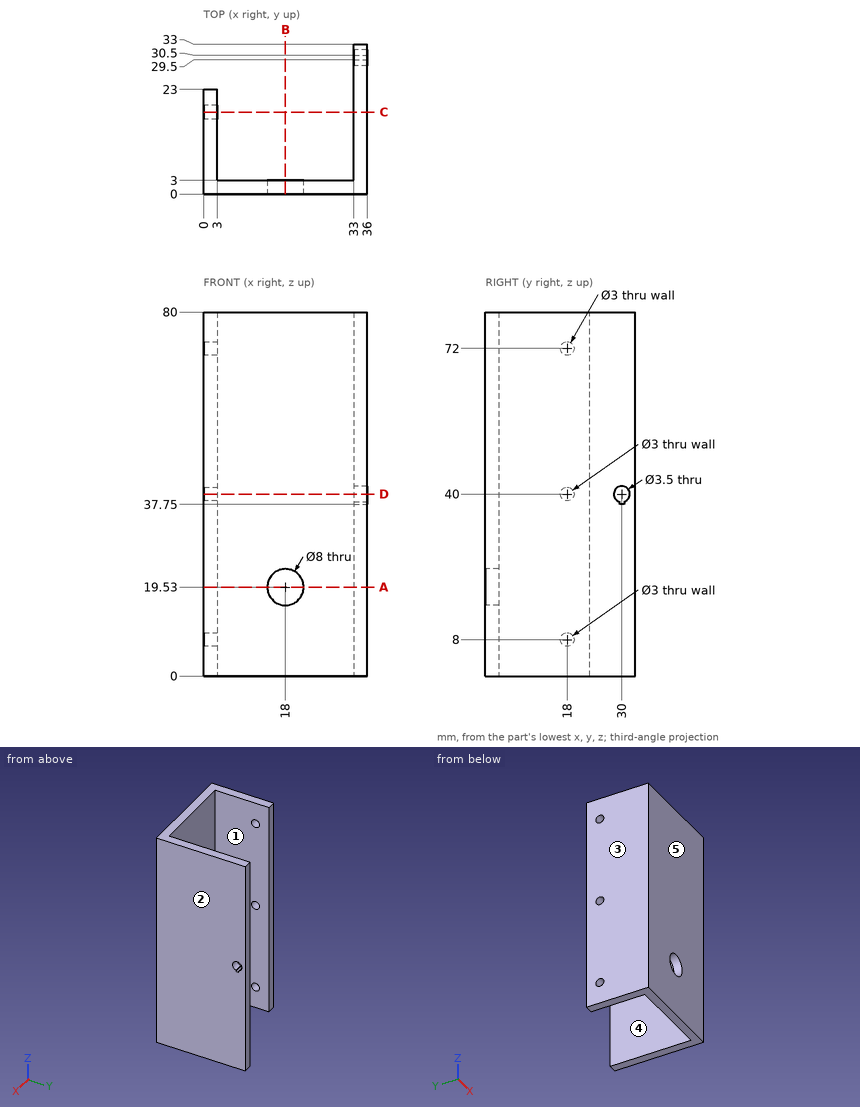
Source: three-view drawing plus pictorial views. Frame: mm from the lowest corner of the part. A direction names the side the tool comes from. Give positions to 0.01 mm unless a question says otherwise; leave off trailing zeros. Order: outer loops, then holes, each group sorted by start corner. A loop starts at its lowest first (then second) coordinate and runs counter-clockwise, first axis right, second up. Notation, with made-up numbers: (77.25, -28) - (106.25, -28) arc R18 ccw to (106.25, 5) - close; hole circle Ø3 at (-28.75, 0.5). An arc over 180 degrees is marked (long way). Put each result on its own line as item: value.
Item 1: Ray query, L1, parallel to X at y = 12, z = 74; L2, parallel to Y at x = 0.95, z = 40; L3, parallel to Z at x = 18, y = 2. Return the intervals inside material, ascending. Write a range as from..to.
Found:
L1: x = 0..3, 33..36
L2: y = 0..16.5, 19.5..23
L3: z = 0..15.53, 23.53..80
Item 2: Contact query for flat-ended pins moving along their axis: pin 1 (2.5 mm diameter, centred on y = 18, z = 72, fed in from -X); pin 2 (9 mm diameter, centred on x = 22, z = 59.5, fed in from +Y); pin 3 (3.5 mm diameter, centred on x = 2, z = 29, fed in from +Y); pin 4 (5 mm diameter, centred on x = 18, z = 19.53, fed in from +Y). Output: stop coordinate, or through.
Found:
pin 1: stops at x = 33
pin 2: stops at y = 3
pin 3: stops at y = 23
pin 4: passes through
Item 3: Section query A-A, the plane z = 19.53. Return loops of the section in (x, y), then the cut area to 3 significant figures.
Found:
outline: (0, 0) - (14, 0) - (14, 3) - (3, 3) - (3, 23) - (0, 23) - close; (22, 0) - (36, 0) - (36, 33) - (33, 33) - (33, 3) - (22, 3) - close
area: 234 mm^2
Item 4: Section query D-D, the plane z = 40. Return loops of the section in (x, y).
Found:
outline: (0, 0) - (36, 0) - (36, 28.25) - (33, 28.25) - (33, 3) - (3, 3) - (3, 16.5) - (0, 16.5) - close; (0, 19.5) - (3, 19.5) - (3, 23) - (0, 23) - close; (33, 31.75) - (36, 31.75) - (36, 33) - (33, 33) - close
Item 5: Section query C-C, the plane y = 18. Return loops of the section in (x, z), then the cut area to 3 significant figures.
Found:
outline: (0, 0) - (3, 0) - (3, 6.5) - (0, 6.5) - close; (0, 9.5) - (3, 9.5) - (3, 38.5) - (0, 38.5) - close; (0, 41.5) - (3, 41.5) - (3, 70.5) - (0, 70.5) - close; (0, 73.5) - (3, 73.5) - (3, 80) - (0, 80) - close; (33, 0) - (36, 0) - (36, 80) - (33, 80) - close
area: 453 mm^2
Item 6: Draft query along X for the marked faces 3, 4 and 5. Return one class per face: +X half, -X half, draft (parallel to the pull), parting line (faces both ways), or undercut.
Found:
face 3: -X half
face 4: undercut
face 5: draft
Item 7: Access query for the marked faces 1 and 2. Directions: +Z, -Z, +X, -X, +Y, -Y. A direction counts if a zero-diameter tool reaches every point of the face in a straight line with its end or side. Return the directions, or none.
Found:
face 1: +Z, -Z, +Y
face 2: +Z, -Z, +X, +Y, -Y
Item 8: Section query B-B, the plane x = 18. Return loops of the section in (y, z), then the cut area to 3 significant figures.
Found:
outline: (0, 0) - (3, 0) - (3, 15.53) - (0, 15.53) - close; (0, 23.53) - (3, 23.53) - (3, 80) - (0, 80) - close
area: 216 mm^2
